```python
from build123d import *

# Parameters (mm, degrees)
F0_R     = 12.5
F1_DEPTH = 10


with BuildPart() as f1:
    # F0 (on Front) → F1 (new body)
    with BuildSketch(Plane.XZ):
        with BuildLine():
            Line((20.260356, 131.683536), (-29.739644, 131.683536))
            Line((-29.739644, 131.683536), (-29.739644, 21.683536))
            Line((-29.739644, 21.683536), (-132.202011, 21.683536))
            ThreePointArc((-132.202011, 21.683536), (-132.236004, 21.471069), (-132.269658, 21.258549))
            Line((-132.269658, 21.258549), (-132.269658, -28.316464))
            Line((-132.269658, -28.316464), (-29.739644, -28.316464))
            Line((-29.739644, -28.316464), (-29.739644, -138.80116))
            Line((-29.739644, -138.80116), (20.260356, -138.80116))
            Line((20.260356, -138.80116), (20.260356, -28.316464))
            Line((20.260356, -28.316464), (133.028674, -28.316464))
            Line((133.028674, -28.316464), (133.028674, 21.683536))
            Line((133.028674, 21.683536), (20.260356, 21.683536))
            Line((20.260356, 21.683536), (20.260356, 131.683536))
        make_face()
        with Locations((-4.739644, -3.316464)):
            Circle(F0_R, mode=Mode.SUBTRACT)
        with BuildLine():
            ThreePointArc((-132.269658, 21.258549), (-132.236004, 21.471069), (-132.202011, 21.683536))
            Line((-132.202011, 21.683536), (-132.269658, 21.683536))
            Line((-132.269658, 21.683536), (-132.269658, 21.258549))
        make_face()
    extrude(amount=F1_DEPTH)


solid = f1.part
```
The listing builds one solid part. Answer for the finished solid, in the listing's coordinates (mm). A direction names the side the tool comes from. Coordinates: 2 decimals unless noted, no trailing zeros. Order: outer loops, then holes, each group sorted by start corner. A loop starts at its lowest first (then second) coordinate and runs counter-clockwise, first axis right, second up. Notation, with made-up numbers: M 40,64.25 L 76,64.25 A11 ccw 76,74.25 Z; hole C -29,47 d8. An arc over 180 degrees is marked long. Answer as a JSON object with one key per item and string values. Group by question number.
1. Determine the mould class of faces 1 (the flat face through (-132.27, -5, -3)), 2 (the flat face through (77, -5, 21.684)), 3 (the cylindrical face through (6.81, -4.93, -8.1)) for opening direction X: released by +X, released by -X, zero draft, split by the parting line, or undercut.
2. Section A-A on x = -6 is taken. Write down the section's boundary in (y, z).
3. Section D-D on z = -95 is taken. Write down the section's boundary in (x, y), then the cut area to 3 significant figures.
4. Section C-C on x = 60 is taken. Write down the section's boundary in (y, z), then the cut area to 3 significant figures.
5. Straight lines are drawn through the part: line 1 (Z direction, x = -5.5, y = -8); line 2 (Z direction, x = 73, y = -7); line 3 (X direction, y = -3.25, z = 68). For each, find the intervals that lie inside material, in ascending order.
6. Flat-ended cylindrical pins translate along their axes: P1, Ø5, axis at x = 49.5, y = -4, coming from the +Z side; P2, Ø2, axis at y = -7, z = -51, coming from the +X side; P3, Ø2, axis at x = 50.5, y = -3, coming from the -Z side; P4, Ø15, axis at x = -4.74, z = -3.32, coming from the +Y side. Find the tip coordinate at first contact, or state that the pin passes through.
7. Section B-B on y = -8.5 is taken. Write down the section's boundary in (x, z), then the cut area to 3 significant figures.
8. A tool of negligible diameter and unlimited length cuts with its end or side. For faces 4 (the flat face through (-80, -5, 21.684)), 5 (the flat face through (76, -5, -28.316)), 6 (the flat face through (-29.74, -5, -83)), from which of +Z, -Z, +X, -X, +Y, -Y can it reach the whole face along a straight path? Write none if from no direction.
Values follow:
{
 "1": {"face 1": "released by -X", "face 2": "zero draft", "face 3": "undercut"},
 "2": {"outline": "M -10,-138.8 L 0,-138.8 L 0,-15.75 L -10,-15.75 Z; M -10,9.12 L 0,9.12 L 0,131.68 L -10,131.68 Z"},
 "3": {"outline": "M -29.74,-10 L 20.26,-10 L 20.26,0 L -29.74,0 Z", "area": "500 mm2"},
 "4": {"outline": "M -10,-28.32 L 0,-28.32 L 0,21.68 L -10,21.68 Z", "area": "500 mm2"},
 "5": {"line 1": "-138.8 to -15.79, 9.16 to 131.68", "line 2": "-28.32 to 21.68", "line 3": "-29.74 to 20.26"},
 "6": {"P1": "z = 21.68", "P2": "x = 20.26", "P3": "z = -28.32", "P4": "through"},
 "7": {"outline": "M -132.27,-28.32 L -29.74,-28.32 L -29.74,-138.8 L 20.26,-138.8 L 20.26,-28.32 L 133.03,-28.32 L 133.03,21.68 L 20.26,21.68 L 20.26,131.68 L -29.74,131.68 L -29.74,21.68 L -132.27,21.68 Z; hole C -4.74,-3.32 d25", "area": "23,800 mm2"},
 "8": {"face 4": "+Z, -X, +Y, -Y", "face 5": "-Z, +X, +Y, -Y", "face 6": "-Z, -X, +Y, -Y"}
}
